Source: CAD feature listing. Evaluate the final solid. Frame: model axes, mm. Round coordinates to 2 decimals unless told otherwise and drop trailing zeros. Loops run counter-clockwise (first coordinate to the right, second up) from the corner with the lowest first, then second, coordinate; pieces in that order, holes last. Notation, with made-up numbers: (-39, 69) - (-25, 69) arc R25 cw to (-25, 92) - close; hole circle Ø4 at (-30, 72). An arc over 180 degrees is marked (long way). Use CSV: the item, a comma, the result in double quotes. Start each with the question number.
from build123d import *

# Parameters (mm, degrees)
F1_DEPTH = 700
F2_R     = 5
F3_DEPTH = 20
F4_R     = 5
F5_DEPTH = 20


with BuildPart() as f1:
    # F0 (on Front) → F1 (new body)
    with BuildSketch(Plane.XZ):
        with BuildLine():
            ThreePointArc((4.5232568237, 2.9976497203), (132.7131971979, 39.9840828273), (260, 0))
            ThreePointArc((260, 0), (133.5510610534, 59.5206573171), (0, 18.3362318665))
            ThreePointArc((0, 18.3362318665), (5.8946060824, 15.8946060824), (8.3362318665, 10))
            ThreePointArc((8.3362318665, 10), (7.3211911397, 6.0134072155), (4.5232568237, 2.9976497203))
        make_face()
        with BuildLine():
            Line((0, 18.3362318665), (0, 1.6637681335))
            ThreePointArc((0, 1.6637681335), (2.3579171095, 2.0041893071), (4.5232568237, 2.9976497203))
            ThreePointArc((4.5232568237, 2.9976497203), (7.3211911397, 6.0134072155), (8.3362318665, 10))
            ThreePointArc((8.3362318665, 10), (5.8946060824, 15.8946060824), (0, 18.3362318665))
        make_face()
        with BuildLine():
            ThreePointArc((0, 18.3362318665), (-8.3362318665, 10), (0, 1.6637681335))
            Line((0, 1.6637681335), (0, 18.3362318665))
        make_face()
    extrude(amount=F1_DEPTH)

    # F2 (on face) → F3 (join)
    with BuildSketch(Plane.XZ.offset(700)):
        with Locations((0, 10)):
            Circle(F2_R)
    extrude(amount=F3_DEPTH)

    # F4 (on face) → F5 (join)
    with BuildSketch(Plane(origin=(0, 0, 0), x_dir=(-1, 0, 0), z_dir=(0, 1, 0))):
        with Locations((0, 10)):
            Circle(F4_R)
    extrude(amount=F5_DEPTH)


solid = f1.part
1. Line query: line 1 along Y through (x, z) = (168, 43); line 2 along X through (y, z) = (-432, 19); line 3 along X through (y, z) = (-86, 15). Output: solid intervals per line, ascending.
2. Section query B-B on x = 36. Return the cut outline in (y, z), and give its area (3 significant figures).
3. Section query C-C on y = -123. Return the cut outline in (x, z).
4. Section query A-A on z = 26.5. Return the cut outline in (x, y).
5. Contact query for flat-ended pins moving along their axis: P1, Ø8, axis at x = 113, y = -156, coming from the +Z side; P2, Ø12, axis at x = 211.5, y = -532, coming from the -Z side; P3, Ø1.5, axis at y = -638, z = 24.5, coming from the -X side. Output: stop coordinate, or through.
Values:
1,line 1,"y = -700 to 0"
1,line 2,"x = 0.84 to 33.71, 226.29 to 239.04"
1,line 3,"x = -6.67 to 25.42, 234.58 to 243.99"
2,outline,"(-700, 20.03) - (0, 20.03) - (0, 40.84) - (-700, 40.84) - close"
2,area,"14,600 mm^2"
3,outline,"(0, 18.34) arc R8.34 ccw (long way) to (4.52, 3) arc R231.25 cw to (260, 0) arc R193.47 ccw to start"
4,outline,"(11.13, -700) - (52.14, -700) - (52.14, 0) - (11.13, 0) - close; (207.86, -700) - (228.75, -700) - (228.75, 0) - (207.86, 0) - close"
5,P1,"stops at z = 59.98"
5,P2,"stops at z = 22.81"
5,P3,"stops at x = 7.19"
